from build123d import *

# Parameters (mm, degrees)
F0_W      = 80
F0_H      = 50
F1_DEPTH  = 2
F2_W      = 75.6
F2_H      = 45.6
F3_DEPTH  = 2
F4_R      = 3
F5_R      = 1.7
F5_R_2    = 1.65
F6_DEPTH  = 25
F7_R      = 4
F7_R_2    = 1.65
F8_DEPTH  = 12
F9_R      = 4
F9_R_2    = 1.7
F10_DEPTH = 10


with BuildPart() as f1:
    # F0 (on Top) → F1 (new body)
    with BuildSketch(Plane.XY):
        Rectangle(F0_W, F0_H)
    extrude(amount=F1_DEPTH)

    # F2 (on face) → F3 (join)
    with BuildSketch(Plane.XY.offset(2)):
        Rectangle(F2_W, F2_H)
    extrude(amount=F3_DEPTH)

    # F4
    f4_edges = [f1.edges().sort_by_distance(p)[0] for p in [
        (-37.8, 22.8, 3),
        (-37.8, -22.8, 3),
        (37.8, 22.8, 3),
        (37.8, -22.8, 3),
    ]]
    fillet(f4_edges, radius=F4_R)

    # F5 (on face) → F6 (cut)
    with BuildSketch(Plane(origin=(0, 0, 0), x_dir=(1, 0, 0), z_dir=(0, 0, -1))):
        with Locations((-20, -10)):
            Circle(F5_R)
        with Locations((9, -15.35)):
            Circle(F5_R_2)
    extrude(amount=-F6_DEPTH, mode=Mode.SUBTRACT)

    # F7 (on face) → F8 (join)
    with BuildSketch(Plane.XY.offset(4)):
        with Locations((9, 15.35)):
            Circle(F7_R)
        with Locations((9, 15.35)):
            Circle(F7_R_2, mode=Mode.SUBTRACT)
    extrude(amount=F8_DEPTH)

    # F9 (on face) → F10 (join)
    with BuildSketch(Plane.XY.offset(4)):
        with Locations((-20, 10)):
            Circle(F9_R)
        with Locations((-20, 10)):
            Circle(F9_R_2, mode=Mode.SUBTRACT)
    extrude(amount=F10_DEPTH)


solid = f1.part
For this review, take the finished solid that the model builds, in its own axes (mm). A direction names the side the tool comes from. Coordinates: 2 decimals unless noted, no trailing zeros. Order: outer loops, then holes, each group sorted by start corner. A loop starts at its lowest first (then second) coordinate and runs counter-clockwise, first axis right, second up. Notation, with made-up numbers: (42, 58) -> (57, 58) arc R14 cw to (57, 84) -> close; hole circle Ø9 at (25, 61). An arc over 180 degrees is marked (long way). Return JSON: item names as keys, results as strings.
1. Machinability: for faces 1 (the flat face through (-3, -24, 2)), 2 (the flat face through (0, -22.8, 3)), 3 (the flat face through (-37.8, 0, 3)), which of the approach directions +Z, -Z, +X, -X, +Y, -Y give a long, thin tool a straight path to every point of the face, cutting with its end or side? Answer none if there is none.
Answer block:
{"face 1": "+Z", "face 2": "+Z, +X, -X, -Y", "face 3": "+Z, -X, +Y, -Y"}
2. For pin 1 Ø0.6 at (y, z) = (-4, 2.5) entering from -X; pin 2 Ø6.5 at (x, y) = (-21, 9.5) entering from +Z; pin 3 Ø1 at (x, z) = (-24, 12.5) entering from +Y, all flat-tipped, find the tip position at first contact; note any pin that passes through.
Answer block:
{"pin 1": "x = -37.8", "pin 2": "z = 14", "pin 3": "y = 11.94"}
3. We need section C-C on z = 10.75. Write out the cut boundary in (x, y).
Answer block:
{"outline": "circle Ø8 at (-20, 10); circle Ø8 at (9, 15.35); hole circle Ø3.4 at (-20, 10); hole circle Ø3.3 at (9, 15.35)"}
4. We need section B-B on x = 9. Write out the cut boundary in (y, z), and give its area (3 significant figures).
Answer block:
{"outline": "(-25, 0) -> (13.7, 0) -> (13.7, 16) -> (11.35, 16) -> (11.35, 4) -> (-22.8, 4) -> (-22.8, 2) -> (-25, 2) -> close; (17, 0) -> (25, 0) -> (25, 2) -> (22.8, 2) -> (22.8, 4) -> (19.35, 4) -> (19.35, 16) -> (17, 16) -> close", "area": "234 mm²"}
5. For line 1 (Y direction, x = 9, z = 7.75); line 2 (Y direction, x = -20, z = 10); line 3 (Z direction, x = -18.5, y = -12), list the stretches that pass through material, from the lowest coordinate up. Write a range as from..to.
Answer block:
{"line 1": "11.35..13.7, 17..19.35", "line 2": "6..8.3, 11.7..14", "line 3": "0..4"}
6. We need section D-D on x = -2. Write out the cut boundary in (y, z).
Answer block:
{"outline": "(-25, 0) -> (25, 0) -> (25, 2) -> (22.8, 2) -> (22.8, 4) -> (-22.8, 4) -> (-22.8, 2) -> (-25, 2) -> close"}
7. The part is to be moulded in two halves that separate along Y. For faces 4 (the flat face through (37.8, 0, 3)), 5 (the cylindrical face through (8.64, 13.74, 7.89)), 6 (the cylindrical face through (-36.9, -21.94, 3.01)), say which applies: +Y half, -Y half, draft (parallel to the pull), parting line (faces both ways), or undercut.
Answer block:
{"face 4": "draft", "face 5": "undercut", "face 6": "-Y half"}
8. We need section A-A on y = 15.35. Write out the cut boundary in (x, z).
Answer block:
{"outline": "(-40, 0) -> (7.35, 0) -> (7.35, 16) -> (5, 16) -> (5, 4) -> (-37.8, 4) -> (-37.8, 2) -> (-40, 2) -> close; (10.65, 0) -> (40, 0) -> (40, 2) -> (37.8, 2) -> (37.8, 4) -> (13, 4) -> (13, 16) -> (10.65, 16) -> close"}
